CAD build for the part. Positions are in the model's coordinates, mm. Face numbers are marked on the shaded views. A direction names the side the tool comes from. Round coordinates to 2 decimals unless told otherwise and drop trailing zeros. Order: outer loops, then holes, each group sorted by start corner. A loop starts at its lowest first (then second) coordinate and runs counter-clockwise, first axis right, second up. Notation, with made-up numbers: (25, 37.5) -> (69, 37.5) arc R33 cw to (69, 66.5) -> close; hole circle Ø2 at (7, 35). An arc over 180 degrees is marked (long way). Answer as CSV lines item,"result". Start each with the question number.
Autodesk Inventor part; units mm, degrees
ref_plane "YZ Plane" through (0, 0, 0) normal (1, 0, 0) x (0, 1, 0)
ref_plane "XZ Plane" through (0, 0, 0) normal (0, 1, 0) x (-1, 0, 0)
ref_plane "XY Plane" through (0, 0, 0) normal (0, 0, 1) x (1, 0, 0)
sketch "Sketch1" plane through (0, 0, 0) normal (0, 0, 1) x (1, 0, 0)
  line L0 (0, 0) -> (100, 0)
  line L1 (100, 0) -> (100, -200)
  line L2 (100, -200) -> (0, -200)
  line L3 (0, -200) -> (0, 0)
  line L4 (100, 0) -> (90, 0)
  line L5 (90, 0) -> (90, -10)
  line L6 (90, -10) -> (100, -10)
  line L7 (100, -10) -> (100, 0)
  line L8 (100, -200) -> (90, -200)
  line L9 (90, -200) -> (90, -190)
  line L10 (90, -190) -> (100, -190)
  line L11 (100, -190) -> (100, -200)
  dimension "d0" = 100
  dimension "d1" = 200
  dimension "d2" = 10
  dimension "d3" = 10
extrude "Plate1" add sketch "Sketch1" along normal blind 3.048 contours L0 L5 L6 L1 L10 L9 L2 L3
sketch "Sketch2" plane through (0, 0, 3.048) normal (0, 0, 1) x (1, 0, 0)
  line L0 (13.9517, -33.0603) -> (49.292, -33.0603) construction
  line L1 (49.292, -33.0603) -> (49.292, -43.4735) construction
  line L2 (49.292, -43.4735) -> (13.9517, -43.4735) construction
  line L3 (13.9517, -43.4735) -> (13.9517, -33.0603) construction
  point P0 (0, 0)
mark "Mark1"
sketch "Sketch3" plane through (3.048, -200, 0) normal (-1, 0, 0) x (0, -1, 0)
  line L0 (-200, 0) -> (0, 0)
  line L1 (0, 0) -> (0, 25)
  line L2 (0, 25) -> (-200, 25)
  line L3 (-200, 25) -> (-200, 0)
edge flange "Flange1" height 25 angle 90 thickness 3.048 bend radius 3.048 thickness toward (-1, 0, 0) relief tear relief width 3.048 relief depth 1.524 edges at (0, -100, 3.048) wall of the first edge with corners at (3.048, 0, 0) (3.048, -200, 0) (3.048, -200, 25) (3.048, 0, 25)
bend "Bend1"
corner "Corner1"
equation "\"d4\" = Thickness"
equation "\"d5\" = BendReliefWidth"
equation "\"d6\" = BendReliefDepth"
equation "\"d7\" = MinimumRemnant"
equation "\"d8\" = TransitionRadius"
equation "\"d11\" = BendRadius"
equation "\"d12\" = CornerReliefSize"
equation "\"d13\" = GapSize"
equation "\"d14\" = JacobiRadiusSize"
equation "\"BendRadius\" = Thickness"
equation "\"BendReliefWidth\" = Thickness"
equation "\"BendReliefDepth\" = 0.5 * Thickness"
equation "\"CornerReliefSize\" = 4 * Thickness"
equation "\"MinimumRemnant\" = 2 * Thickness"
equation "\"TransitionRadius\" = BendRadius"
equation "\"JacobiRadiusSize\" = BendRadius"
equation "\"GapSize\" = Thickness"
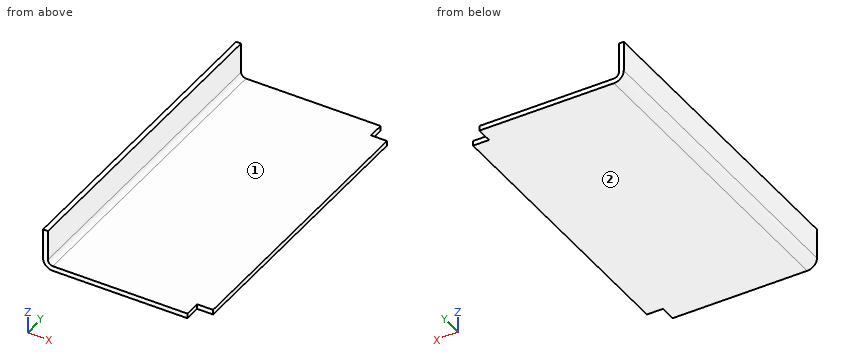
Item 1: Probe line 1 (Z direction, x = 29, y = -134); line 2 (X direction, y = -110.5, z = 2). List the from-to ranges inside material, lowest first.
Item 2: Band-saw the part on C-C, the plane z = 18. Give the cut face in (x, y), and give its area (3 significant figures).
Item 3: Band-saw the part on A-A, the plane y = -81.5. Give the cut face in (x, z).
Item 4: Pin check, flat tips, straight feed: pin 1 (2.5 mm diameter, centred on x = 96.5, z = 1.5, fed in from +Y); pin 2 (1.5 mm diameter, centred on x = 93, z = 1.5, fed in from -Y); pin 3 (2.5 mm diameter, centred on y = -4.5, z = 2, fed in from +X). Stop position of each tip, or through.
Item 5: Band-saw the part on B-B, the plane x = 93.5. Give the cut face in (y, z), and give its area (3 significant figures).
Item 6: Tool access for the marked faces 1 and 2: list every direction of +Z, -Z, +X, -X, +Y, -Y with a clear straight run to the whole face (end or side of a thin tool).
Values:
1,line 1,"0 to 3.05"
1,line 2,"1.58 to 100"
2,outline,"(0, -200) -> (3.05, -200) -> (3.05, 0) -> (0, 0) -> close"
2,area,"610 mm²"
3,outline,"(0, 6.1) arc R6.1 ccw to (6.1, 0) -> (100, 0) -> (100, 3.05) -> (6.1, 3.05) arc R3.05 cw to (3.05, 6.1) -> (3.05, 25) -> (0, 25) -> close"
4,pin 1,"y = -10"
4,pin 2,"y = -190"
4,pin 3,"x = 90"
5,outline,"(-190, 0) -> (-10, 0) -> (-10, 3.05) -> (-190, 3.05) -> close"
5,area,"549 mm²"
6,face 1,"+Z, +X, +Y, -Y"
6,face 2,"-Z, +X, -X, +Y, -Y"
